CAD build for the part. Positions are in the model's coordinates, mm. A direction names the side the tool comes from. Coordinates: 2 decimals unless noted, no trailing zeros. Loops run counter-clockwise (first coordinate to the right, second up) from the corner with the lowest first, then second, coordinate; pieces in that order, holes last. Notation, with made-up numbers: (-20.5, 52) -> (3.5, 52) arc R25 cw to (3.5, 76) -> close; hole circle Ø4 at (78.25, 15). An arc over 180 degrees is marked (long way). Answer as CSV lines item,"result". Start each with the question number.
from build123d import *

# Parameters (mm, degrees)
SKETCH1_W           = 30
SKETCH1_H           = 7
BOSS_EXTRUDE1_DEPTH = 23.5
BOSS_EXTRUDE2_DEPTH = 10.8


with BuildPart() as part:
    # Sketch1 → Boss-Extrude1 (new, symmetric)
    with BuildSketch(Plane.XY):
        Polygon((7.5, 7), (7.5, -2.4), (15, -2.4), (15, 9), (-15, 9), (-15, -2.4), (-7.5, -2.4), (-7.5, 7), align=None)
        with Locations((0, 12.5)):
            Rectangle(SKETCH1_W, SKETCH1_H)
    extrude(amount=BOSS_EXTRUDE1_DEPTH, both=True)

    # Sketch1_3 → Boss-Extrude2 (add, symmetric)
    with BuildSketch(Plane.XY):
        Polygon((15, 16), (15, 9), (23.5, 9), (23.5, 17), (-23.5, 17), (-23.5, 9), (-15, 9), (-15, 16), align=None)
    extrude(amount=BOSS_EXTRUDE2_DEPTH, both=True)


solid = part.part
Item 1: Wall check: probe 1 along X at (y, z) = (1, 21); probe 2 along X at (y, z) = (14.75, -11); probe 3 along Z at (x, y) = (-19, 12.75). Give the ranges that are in metal, low to high.
Item 2: Flat gauge pins, fed straight in: pin 1 Ø10 at (x, z) = (-5, 18.5) entering from +Y; pin 2 Ø2.5 at (x, z) = (-19, 2) entering from -Y; pin 3 Ø1 at (y, z) = (6, -11) entering from -X. Where does each tip first touch, or does it go through?
Item 3: Which spindle directions (+Z, -Z, +X, -X, +Y, -Y) get a long thin tool onto all of the face, cutting with end or side? Do faces 1 (the face through (-19, 9, 0)), 2 (the face through (0, 7, 0)), 3 (the face through (0, 16, -17)). Say none if no direction does.
Item 4: Saw through at D-D (y = 12). Write the cut outline in (x, z).
Item 5: Saw through at C-C (z = -8.5). Write the cut outline in (x, y), plus the area to 3 significant figures.
Item 6: Saw through at B-B (x = 11.5). Write the cut outline in (y, z), plus the area to 3 significant figures.
Item 7: Saw through at A-A (y = 5). Write the cut outline in (x, z), plus the area to 3 significant figures.
Geometry check:
1,probe 1,"-15 to -7.5, 7.5 to 15"
1,probe 2,"-15 to 15"
1,probe 3,"-10.8 to 10.8"
2,pin 1,"y = 16"
2,pin 2,"y = 9"
2,pin 3,"x = -15"
3,face 1,"+Z, -Z, -X, -Y"
3,face 2,"+Z, -Z, -Y"
3,face 3,"-Z, +X, -X, +Y"
4,outline,"(-23.5, -10.8) -> (-15, -10.8) -> (-15, -23.5) -> (15, -23.5) -> (15, -10.8) -> (23.5, -10.8) -> (23.5, 10.8) -> (15, 10.8) -> (15, 23.5) -> (-15, 23.5) -> (-15, 10.8) -> (-23.5, 10.8) -> close"
5,outline,"(-23.5, 9) -> (-15, 9) -> (-15, -2.4) -> (-7.5, -2.4) -> (-7.5, 7) -> (7.5, 7) -> (7.5, -2.4) -> (15, -2.4) -> (15, 9) -> (23.5, 9) -> (23.5, 17) -> (-23.5, 17) -> close"
5,area,"577 mm2"
6,outline,"(-2.4, -23.5) -> (16, -23.5) -> (16, -10.8) -> (17, -10.8) -> (17, 10.8) -> (16, 10.8) -> (16, 23.5) -> (-2.4, 23.5) -> close"
6,area,"886 mm2"
7,outline,"(-15, -23.5) -> (-7.5, -23.5) -> (-7.5, 23.5) -> (-15, 23.5) -> close; (7.5, -23.5) -> (15, -23.5) -> (15, 23.5) -> (7.5, 23.5) -> close"
7,area,"705 mm2"
